Here's the drawing with two shaded views (mm, measured from the low corner). I have some questions. A direction names the side the tool comes from. Round coordinates to 2 decimals unless told otherwise and drop trailing zeros. Write each loop counter-clockwise with the first axis right and the second up, starting at its lowest first coordinate (ties: lowest second). Pieces come first, ordered by that corner, then holes. Notation, with made-up numbers: M 32,78 L 65,78 A32 ccw 65,111 Z; hole C 58,80.5 d1. An arc over 180 degrees is marked long. Write item = value, one per line. Start each with the question number.
(1) Will these pins go through, and if not, where does the flat tip stop? pin 1 Ø2 at (x, y) = (8.5, 2.5) entering from +Z; pin 2 Ø1 at (x, z) = (10.5, 11) entering from -Y; pin 3 Ø1 at (x, y) = (8.5, 1.5) entering from -Z; pin 4 Ø1 at (y, z) = (4.5, 5.5) entering from +X.
(2) I want a section at A-A (y = 1.45). List the corners of the cut face in (x, z) for me, and give its area (3 significant figures).
(3) If we mould it in two halves opening along Z, with no side actions, what happens to the marked faces 3 and 4? For each: released by +Z, released by -Z, zero draft, split by the parting line, or undercut.
(4) I need wall thicknesses on line 1 along Z through (x, y) = (9.5, 3.2); line 2 along Z through (x, y) = (9.5, 5.6); line 3 along Y through (x, z) = (1.25, 10.5). Which ranges of each line are inside material? Lowest first, please.
(5) On a 3-axis mill with a long thin cutter (end or side, diameter ignored), from which of +Z, -Z, +X, -X, +Y, -Y can I reach the whole of each face in a straight line? I mean the marked faces 1 and 2. Say none if no direction works.
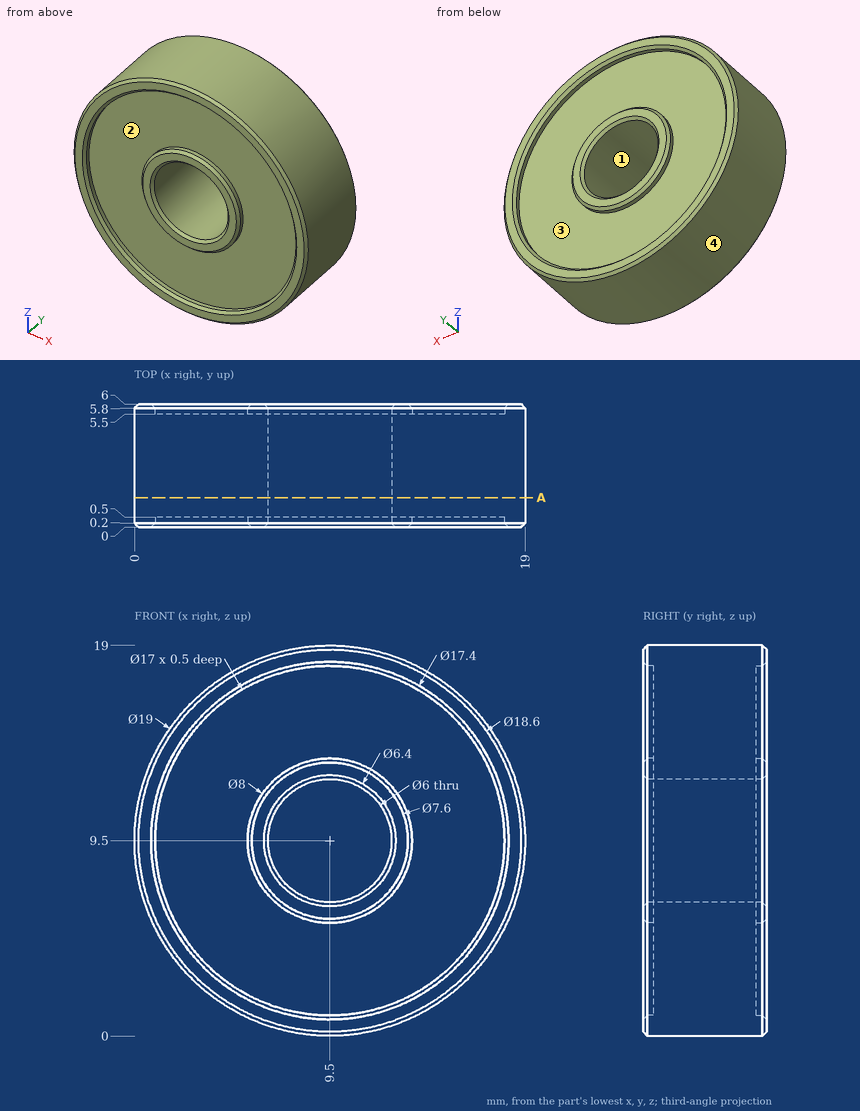
Returned:
q1.pin_1 = 19
q1.pin_2 = through
q1.pin_3 = 0.01
q1.pin_4 = 18.33
q2.outline = C 9.5,9.5 d19; hole C 9.5,9.5 d6
q2.area = 255 mm²
q3.face_3 = undercut
q3.face_4 = split by the parting line
q4.line_1 = 0 to 6.5, 12.5 to 19
q4.line_2 = 0 to 1, 5.5 to 6.5, 12.5 to 13.5, 18 to 19
q4.line_3 = 0.5 to 5.5
q5.face_1 = +Y, -Y
q5.face_2 = -Y
